from build123d import *

# Parameters (mm, degrees)
BOSS_EXTRUDE1_DEPTH = 55
SKETCH2_W           = 0.5
SKETCH2_H           = 4.754059282
SKETCH2_H_2         = 4.044844813
CUT_EXTRUDE1_DEPTH  = 2.25


with BuildPart() as part:
    # Sketch1 → Boss-Extrude1 (new body)
    with BuildSketch(Plane(origin=(0, 0, 0), x_dir=(0, 0, -1), z_dir=(1, 0, 0))):
        with BuildLine():
            Line((12.38, 0.625), (-12.38, 0.625))
            ThreePointArc((-12.38, 0.625), (-12.818406204, 0.443406204), (-13, 0.005))
            Line((-13, 0.005), (-13, -0.005))
            ThreePointArc((-13, -0.005), (-12.818406204, -0.443406204), (-12.38, -0.625))
            Line((-12.38, -0.625), (12.38, -0.625))
            ThreePointArc((12.38, -0.625), (12.818406204, -0.443406204), (13, -0.005))
            Line((13, -0.005), (13, 0.005))
            ThreePointArc((13, 0.005), (12.818406204, 0.443406204), (12.38, 0.625))
        make_face()
    extrude(amount=BOSS_EXTRUDE1_DEPTH)

    # Sketch2 → Cut-Extrude1 (cut, through all)
    with BuildSketch(Plane(origin=(0, 0.625, 0), x_dir=(1, 0, 0), z_dir=(0, 1, 0))):
        with BuildLine():
            ThreePointArc((15.382256297, 3.997225745), (15.367075517, -0.996463715), (15.882256297, 3.97060319))
            Line((15.882256297, 3.97060319), (15.882256297, 12.38))
            Line((15.882256297, 12.38), (15.382256297, 12.38))
            Line((15.382256297, 12.38), (15.382256297, 3.997225745))
        make_face()
        with BuildLine():
            Line((42.746308765, 12.38), (42.246308765, 12.38))
            Line((42.246308765, 12.38), (42.246308765, 3.987094843))
            ThreePointArc((42.246308765, 3.987094843), (42.50370983, -0.999997247), (42.746308765, 3.98783681))
            Line((42.746308765, 3.98783681), (42.746308765, 12.38))
        make_face()
        with Locations((15.632256297, 14.757029641)):
            Rectangle(SKETCH2_W, SKETCH2_H)
        with Locations((42.496308765, 14.402422407)):
            Rectangle(SKETCH2_W, SKETCH2_H_2)
    extrude(amount=-CUT_EXTRUDE1_DEPTH, mode=Mode.SUBTRACT)


solid = part.part
Design review of the part built by this model. Coordinates are the model's own, in mm. A direction names the side the tool comes from. Coordinates: 2 decimals unless noted, no trailing zeros. Write each loop counter-clockwise with the first axis right and the second up, starting at its lowest first coordinate (ties: lowest second). Pieces come first, ordered by that corner, then holes. Notation, with made-up numbers: (78.5, 77) -> (122.5, 77) arc R11 ccw to (122.5, 81) -> close; hole circle Ø7 at (3.25, 42.25). An arc over 180 degrees is marked (long way). Write each question's results on one line, items separated by ' | '. Start each with the question number.
(1) Take a section at A-A on z = -1.5. Write out the cut boundary in (x, y) (3 decimals), and give its area (4 significant figures).
(2) Tool access review of faces 4 (the face through (15.882, 0, -8)), 5 (the face through (27, -0.625, 0)): name each direction out of +Z, -Z, +X, -X, +Y, -Y from which nothing blocks a thin tool from reaching the whole face with its end or side.
(3) For line 1 along X through (y, z) = (0.3, -1.5); line 2 along X through (y, z) = (-0.25, -9.5); line 3 along Z through (x, y) = (42.5, -0.05), list the stretches that pass through material, from the lowest coordinate up. Write a range as from..to.
(4) Clearance check with a flat-ended pin moving along its axis: P1, Ø3, axis at x = 42.5, z = -1.5, coming from the -Y side. State where the tip first meets the part, or that it passes through.
(5) The part is to be moulded in two halves that separate along Z. For faces 1 (the face through (42.4, 0, 1)), 2 (the face through (15.382, 0, -9)), 3 (the face through (15.26, 0.01, 0.99)), say which applies: pulls with the +Z half, pulls with the -Z half, needs draft (parallel to the pull), parting line crosses it, or undercut.
(6) Take a section at B-B on y = 0.4. Write out the cut boundary in (x, z), and give its area (3 significant figures).
Results found:
1) outline: (0, -0.625) -> (13, -0.625) -> (13, 0.625) -> (0, 0.625) -> close; (18, -0.625) -> (40, -0.625) -> (40, 0.625) -> (18, 0.625) -> close; (45, -0.625) -> (55, -0.625) -> (55, 0.625) -> (45, 0.625) -> close | area: 56.25 mm2
2) face 4: -Z, +Y, -Y | face 5: +Z, -Z, +X, -X, -Y
3) line 1: x = 0..13, 18..40, 45..55 | line 2: x = 0..15.38, 15.88..42.25, 42.75..55 | line 3: z = 1..13
4) P1: passes through
5) face 1: undercut | face 2: needs draft | face 3: undercut
6) outline: (0, -12.86) -> (15.38, -12.86) -> (15.38, -4) arc R2.5 cw (long way) to (15.88, -3.97) -> (15.88, -12.86) -> (42.25, -12.86) -> (42.25, -3.99) arc R2.5 cw (long way) to (42.75, -3.99) -> (42.75, -12.86) -> (55, -12.86) -> (55, 12.86) -> (0, 12.86) -> close | area: 1,370 mm2
